```python
from build123d import *

# Parameters (mm, degrees)
F0_W         = 142.24
F0_H         = 71.12
F1_DEPTH     = 12.192
F3_T         = -4.826
F4_D         = 12.192
F5_R         = 6.1468
F6_T1_DEPTH  = 129.9464
F6_T3_DEPTH  = 58.8264
F6_T6_ANGLE  = 90
F6_T8_ANGLE  = 90
F6_T10_ANGLE = 90
F6_T12_ANGLE = 90
F7_R         = 5.08


# Not quite as in the source:
# - a fillet or chamfer that OpenCascade refuses, or shapes differently, is made with other operations: its cross-section is extruded or revolved along the edge and cut away or added
# - a feature names something its author has since deleted; it is built from what else it names


with BuildPart() as f1:
    # F0 (on Top) → F1 (new body)
    with BuildSketch(Plane.XY):
        Rectangle(F0_W, F0_H)
    extrude(amount=F1_DEPTH)

    # F3
    f3_openings = [f1.faces().sort_by_distance(p)[0] for p in [
        (0, 0, 0),
    ]]
    offset(amount=F3_T, openings=f3_openings)

    # F4 (through all)
    with Locations(Plane(origin=(0, 0, 0), x_dir=(1, 0, 0), z_dir=(0, 0, -1))):
        with Locations((59.7701932977, -12.9658412188), (59.7701932977, -23.8187816803)):
            Hole(F4_D / 2)

    # F5
    f5_edges = [f1.edges().sort_by_distance(p)[0] for p in [
        (66.294, -30.734, 3.683),
        (66.294, 30.734, 3.683),
        (-66.294, 30.734, 3.683),
        (-66.294, -30.734, 3.683),
        (-71.12, 35.56, 6.096),
        (-71.12, -35.56, 6.096),
        (71.12, -35.56, 6.096),
        (71.12, 35.56, 6.096),
    ]]
    fillet(f5_edges, radius=F5_R)

    # F6: fillet of radius 5.08 on 1 edges, made by hand

    # F6_s2 → F6_t1 (cut)
    with BuildSketch(Plane.YZ.offset(-64.9732)):
        with BuildLine():
            ThreePointArc((30.48, 0), (34.0721024484, 1.4878975516), (35.56, 5.08))
            Line((35.56, 5.08), (35.56, 0))
            Line((35.56, 0), (30.48, 0))
        make_face()
        with BuildLine():
            ThreePointArc((-35.56, 5.08), (-34.0721024484, 1.4878975516), (-30.48, 0))
            Line((-30.48, 0), (-35.56, 0))
            Line((-35.56, 0), (-35.56, 5.08))
        make_face()
    extrude(amount=F6_T1_DEPTH, mode=Mode.SUBTRACT)

    # F6_s4 → F6_t3 (cut)
    with BuildSketch(Plane.XZ.offset(-29.4132)):
        with BuildLine():
            ThreePointArc((-66.04, 0), (-69.6321024484, 1.4878975516), (-71.12, 5.08))
            Line((-71.12, 5.08), (-71.12, 0))
            Line((-71.12, 0), (-66.04, 0))
        make_face()
        with BuildLine():
            ThreePointArc((66.04, 0), (69.6321024484, 1.4878975516), (71.12, 5.08))
            Line((71.12, 5.08), (71.12, 0))
            Line((71.12, 0), (66.04, 0))
        make_face()
    extrude(amount=F6_T3_DEPTH, mode=Mode.SUBTRACT)

    # F6_s5 → F6_t6 (revolve, cut)
    with BuildSketch(Plane.XZ.offset(-29.4132)):
        with BuildLine():
            ThreePointArc((66.04, 0), (69.6321024484, 1.4878975516), (71.12, 5.08))
            Line((71.12, 5.08), (71.12, 0))
            Line((71.12, 0), (66.04, 0))
        make_face()
    revolve(axis=Axis((64.9732, 29.4132, 0), (0, 0, 1)), revolution_arc=F6_T6_ANGLE, mode=Mode.SUBTRACT)

    # F6_s7 → F6_t8 (revolve, cut)
    with BuildSketch(Plane.XZ.offset(-29.4132)):
        with BuildLine():
            ThreePointArc((-66.04, 0), (-69.6321024484, 1.4878975516), (-71.12, 5.08))
            Line((-71.12, 5.08), (-71.12, 0))
            Line((-71.12, 0), (-66.04, 0))
        make_face()
    revolve(axis=Axis((-64.9732, 29.4132, 0), (0, 0, -1)), revolution_arc=F6_T8_ANGLE, mode=Mode.SUBTRACT)

    # F6_s9 → F6_t10 (revolve, cut)
    with BuildSketch(Plane.YZ.offset(-64.9732)):
        with BuildLine():
            ThreePointArc((-30.48, 0), (-34.0721024484, 1.4878975516), (-35.56, 5.08))
            Line((-35.56, 5.08), (-35.56, 0))
            Line((-35.56, 0), (-30.48, 0))
        make_face()
    revolve(axis=Axis((-64.9732, -29.4132, 0), (0, 0, -1)), revolution_arc=F6_T10_ANGLE, mode=Mode.SUBTRACT)

    # F6_s11 → F6_t12 (revolve, cut)
    with BuildSketch(Plane.YZ.offset(64.9732)):
        with BuildLine():
            ThreePointArc((-30.48, 0), (-34.0721024484, 1.4878975516), (-35.56, 5.08))
            Line((-35.56, 5.08), (-35.56, 0))
            Line((-35.56, 0), (-30.48, 0))
        make_face()
    revolve(axis=Axis((64.9732, -29.4132, 0), (0, 0, 1)), revolution_arc=F6_T12_ANGLE, mode=Mode.SUBTRACT)

    # F7
    f7_edges = [f1.edges().sort_by_distance(p)[0] for p in [
        (0, 35.56, 12.192),
        (69.319644, -33.759644, 12.192),
        (0, -35.56, 12.192),
        (-69.319644, -33.759644, 12.192),
        (-71.12, 0, 12.192),
        (71.12, 0, 12.192),
        (-69.319644, 33.759644, 12.192),
        (69.319644, 33.759644, 12.192),
    ]]
    fillet(f7_edges, radius=F7_R)


solid = f1.part
```
Verification items for the finished model (mm, model axes). A direction names the side the tool comes from. Give positions to 0.01 mm unless a question says otherwise; leave off trailing zeros. Write each loop counter-clockwise with the first axis right and the second up, starting at its lowest first coordinate (ties: lowest second). Pieces come first, ordered by that corner, then holes. Notation, with made-up numbers: M 60,32.25 L 96,32.25 A25 ccw 96,49.25 Z; hole C 4,26 d5. An arc over 180 degrees is marked long. One line per question, with ' | ' between items.
1) Set-up check for faces 4 (the cylindrical face through (60, 29.91, 9.81)), 5 (the cylindrical face through (64.446, 28.981, 3.631)): record each of +Z, -Z, +X, -X, +Y, -Y from which the full face is reachable in a straight line by a thin tool's end or side.
Result:
face 4: +Z, -Z | face 5: -Z
2) Section check A-A on y = 11. Enter the section's corners in (x, z).
Result:
outline: M -71.12,5.08 A5.08 ccw -66.29,0.01 L -66.29,7.37 L 54,7.37 L 54,12.19 L -66.04,12.19 A5.08 ccw -71.12,7.11 Z; M 65.54,7.37 L 66.29,7.37 L 66.29,0.01 A5.08 ccw 71.12,5.08 L 71.12,7.11 A5.08 ccw 66.04,12.19 L 65.54,12.19 Z
3) Mould release check, pull along X, two halves, no side actions. Record for faces 1 (the cylindrical face through (69.37, 33.71, 6.11)), 2 (the cylindrical face through (0.91, 34.032, 10.743)), 3 (the flat face through (-66.294, 0, 4)): released by +X, released by -X, zero draft, split by the parting line, or undercut.
Result:
face 1: released by +X | face 2: zero draft | face 3: undercut
4) Thickness scan on line 1 along X through (y, z) = (10, 5.5); line 2 along Y through (x, z) = (54.5, 5.5); line 3 along Z through (x, y) = (22, -19). Record the ranges inside material, lowest first. Write a range as [from, to].
Result:
line 1: x = [-71.12, -66.29], [66.29, 71.12] | line 2: y = [-35.56, -30.73], [30.73, 35.56] | line 3: z = [7.37, 12.19]
5) Section check B-B on x = -25.5. Enter the section's corners in (y, z).
Result:
outline: M -35.56,5.08 A5.08 ccw -30.73,0.01 L -30.73,7.37 L 30.73,7.37 L 30.73,0.01 A5.08 ccw 35.56,5.08 L 35.56,7.11 A5.08 ccw 30.48,12.19 L -30.48,12.19 A5.08 ccw -35.56,7.11 Z
6) Gauge pin test, flat ends, axial feed: pin 1 Ø1.5 at (x, y) = (25.5, -12.5) entering from -Z; pin 2 Ø2 at (x, z) = (-8, 2) entering from -Y; pin 3 Ø16 at (x, y) = (59.77, 12.97) entering from -Z. Record the tip position at first contact, or that the pin passes through.
Result:
pin 1: stops at z = 7.37 | pin 2: stops at y = -35.11 | pin 3: stops at z = 0.01
7) Section check C-C on y = -11.5. Enter the section's corners in (x, z).
Result:
outline: M -71.12,5.08 A5.08 ccw -66.29,0.01 L -66.29,7.37 L 66.29,7.37 L 66.29,0.01 A5.08 ccw 71.12,5.08 L 71.12,7.11 A5.08 ccw 66.04,12.19 L -66.04,12.19 A5.08 ccw -71.12,7.11 Z
